Input: part model. Units: mm. Frame: model coordinates. Coordinates: 2 decimals unless noted, no trailing zeros. Loops run counter-clockwise (first coordinate to the right, second up) from the corner with the lowest first, then second, coordinate; pieces in that order, holes last.
(1) Contact query for flat-ended pins moving along their axis: P1, Ø1, axis at x = 0.5, y = 89, coming from the -Z side; P2, Ø0.7, axis at x = 1, y = 159, coming from the +Z side; P3, Ø1, axis at x = 0.5, z = 2, coming from the +Y side. Output: stop coordinate, or through.
(2) Section A-A, the plane y = 282.55. Return loops of the section in (x, z) (3 decimals).
(3) Section B-B, the plane x = 1.25. Return loops of the section in (y, z) (3 decimals), then the cut area to 3 significant figures.
(4) Line query: L1, parallel to Z at x = 1.85, y = 282.55 (3 decimals); L2, parallel to Y at x = 1.3, z = -1 (3 decimals); L3, parallel to Y at x = 1.1, z = -0.5. Output: solid intervals per line, ascending.
(5) Section C-C, the plane y = 243. Return loops of the section in (x, z).
Autodesk Inventor part; units mm, degrees
ref_plane "YZ Plane" through (0, 0, 0) normal (1, 0, 0) x (0, 1, 0)
ref_plane "XZ Plane" through (0, 0, 0) normal (0, 1, 0) x (-1, 0, 0)
ref_plane "XY Plane" through (0, 0, 0) normal (0, 0, 1) x (1, 0, 0)
sketch "Sketch4" plane through (0, 0, 0) normal (1, 0, 0) x (0, 1, 0)
  line L0 (0, 0) -> (280, 0)
  line L1 (280, 0) -> (280, -2)
  line L2 (280, -2) -> (0, -2)
  line L3 (0, -2) -> (0, 0)
  circle A0 centre (282.55, -1) radius 2.625
  circle A1 centre (282.55, -1) radius 4.5
  point P0 (278.1625, -2)
  point P1 (278.1625, 0)
  dimension "d10" = 280
  dimension "d11" = 2
  dimension "d12" = 5.25
  dimension "d13" = 9
extrude "Extrusion2" add sketch "Sketch4" along normal blind 2.4 contours L0 A1 L2 L3 | A1 L2 L1 A0 L0 | L0 L1 A0 L2 A1
sketch "Sketch6" plane through (0, 0, -2) normal (0, -1, 0) x (1, 0, 0)
  line L0 (0, 2) -> (0, 0)
  line L1 (0, 0) -> (2.4, 0)
  line L2 (2.4, 0) -> (2.4, 2)
  line L3 (2.4, 2) -> (0, 2)
  line L4 (0, 2) -> (0, 0)
extrude "Extrusion4" add sketch "Sketch6" along normal blind 5
properties part number "guide"
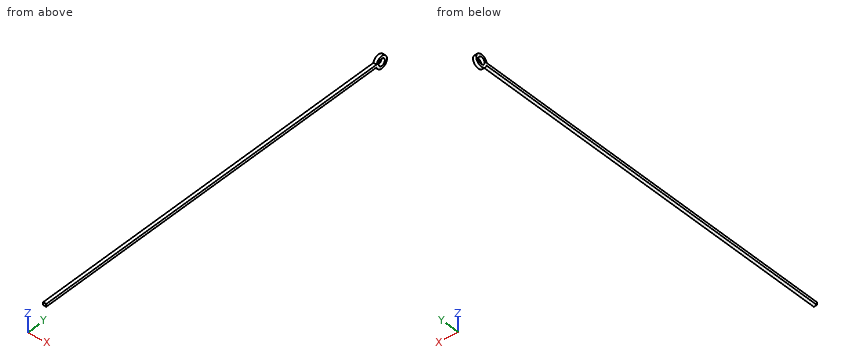
Report:
1. P1: stops at z = -2
1. P2: stops at z = 0
1. P3: stops at y = 286.29
2. outline: (0, -5.5) - (2.4, -5.5) - (2.4, -3.625) - (0, -3.625) - close; (0, 1.625) - (2.4, 1.625) - (2.4, 3.5) - (0, 3.5) - close
3. outline: (-5, -2) - (278.163, -2) arc R4.5 ccw (long way) to (278.163, 0) - (-5, 0) - close; hole circle Ø5.25 at (282.55, -1)
3. area: 608 mm2
4. L1: z = -5.5 to -3.625, 1.625 to 3.5
4. L2: y = -5 to 279.925, 285.175 to 287.05
4. L3: y = -5 to 279.97, 285.13 to 287.02
5. outline: (0, -2) - (2.4, -2) - (2.4, 0) - (0, 0) - close
